Part model, mm, in its own coordinate system. A direction names the side the tool comes from. Round coordinates to 2 decimals unless told otherwise and drop trailing zeros. Write each loop counter-clockwise with the first axis right and the second up, starting at its lowest first coordinate (ties: lowest second). Pieces come first, ordered by that corner, then holes. Notation, with made-up numbers: M 54.5,-5.5 L 103.5,-5.5 A13 cw 103.5,13.5 Z; hole C 54,42.25 d1. An arc over 180 degrees is marked long. Use a Markdown table: item, result. Add a question column.
1) Slice it at D-D on x = 13.5. Write the cut outline in (y, z).
2) Which spindle directions (+Z, -Z, +X, -X, +Y, -Y) get a long thin tool onto all of the face, cutting with end or side? Do faces 1 (the face through (-13, 0, 1.588)), 2 (the face through (38.1, 0, 0)), 3 (the face through (18.78, 2.52, 0.33)). Say none if no direction does.
3) Slice it at A-A on y = 0. Write the cut outline in (x, z), plus the area to 3 significant figures.
4) Two-plate mould, pull along X, no slides. Class faces 4 (the face through (0, 3, 0)), 5 (the face through (-19.05, 0, -2)), 6 (the face through (-9.39, -1.46, -3.52)): released by +X, released by -X, zero draft, split by the parting line, or undercut.
5) Wall check: probe 1 along X at (y, z) = (-2, 0.75); probe 2 along X at (y, z) = (2, -3); probe 3 along Z at (x, y) = (31, -0.25). Give the ranges that are in metal, low to high.
6) Slice it at B-B on x = -15. Write the cut outline in (y, z).
7) Slice it at C-C on z = 0. Write the cut outline in (x, y).
8) Drop flat-ended pins along their axis: P1, Ø2, axis at x = -14, y = 1.5, coming from the -Z side; P2, Ø2, axis at x = -8, y = 2, coming from the -Z side; P3, Ø1.5, axis at x = 3, y = 2.5, coming from the +Z side. Give the stop position or say it passes through.
```python
from build123d import *

# Parameters (mm, degrees)
SKETCH1_R               = 2.54
BOSS_EXTRUDE1_DEPTH     = 38.1
SKETCH2_R               = 3.81
BOSS_EXTRUDE2_DEPTH     = 19.05
SKETCH3_W               = 12.7
SKETCH3_H               = 3.175
CUT_EXTRUDE1_DEPTH      = 4.81
CUT_EXTRUDE1_DEPTH_BACK = 4.81


with BuildPart() as part:
    # Sketch1 → Boss-Extrude1 (new body)
    with BuildSketch(Plane(origin=(0, 0, 0), x_dir=(0, 0, -1), z_dir=(1, 0, 0))):
        Circle(SKETCH1_R)
    extrude(amount=BOSS_EXTRUDE1_DEPTH)

    # Sketch2 → Boss-Extrude2 (add)
    with BuildSketch(Plane(origin=(0, 0, 0), x_dir=(0, 0, -1), z_dir=(1, 0, 0))):
        Circle(SKETCH2_R)
    extrude(amount=-BOSS_EXTRUDE2_DEPTH)

    # Sketch3 → Cut-Extrude1 (cut, two sides)
    with BuildSketch(Plane(origin=(0, 0, 0), x_dir=(1, 0, 0), z_dir=(0, 1, 0))) as cut_extrude1_sk:
        with Locations((-12.7, 0)):
            Rectangle(SKETCH3_W, SKETCH3_H)
    extrude(amount=CUT_EXTRUDE1_DEPTH, mode=Mode.SUBTRACT)
    extrude(cut_extrude1_sk.sketch, amount=-CUT_EXTRUDE1_DEPTH_BACK, mode=Mode.SUBTRACT)


solid = part.part
```
Entries:
| question | item | result |
|---|---|---|
| 1 | outline | C 0,0 d5.08 |
| 2 | face 1 | -X, +Y, -Y |
| 2 | face 2 | +Z, -Z, +X, +Y, -Y |
| 2 | face 3 | +X |
| 3 | outline | M -19.05,-3.81 L 0,-3.81 L 0,-2.54 L 38.1,-2.54 L 38.1,2.54 L 0,2.54 L 0,3.81 L -19.05,3.81 L -19.05,1.59 L -6.35,1.59 L -6.35,-1.59 L -19.05,-1.59 Z |
| 3 | area | 298 mm^2 |
| 4 | face 4 | released by +X |
| 4 | face 5 | released by -X |
| 4 | face 6 | zero draft |
| 5 | probe 1 | x = -6.35 to 38.1 |
| 5 | probe 2 | x = -19.05 to 0 |
| 5 | probe 3 | z = -2.53 to 2.53 |
| 6 | outline | M -3.46,-1.59 A3.81 ccw 3.46,-1.59 Z; M -3.46,1.59 L 3.46,1.59 A3.81 ccw Z |
| 7 | outline | M -6.35,-3.81 L 0,-3.81 L 0,-2.54 L 38.1,-2.54 L 38.1,2.54 L 0,2.54 L 0,3.81 L -6.35,3.81 Z |
| 8 | P1 | stops at z = -3.78 |
| 8 | P2 | stops at z = -3.68 |
| 8 | P3 | stops at z = 1.84 |
